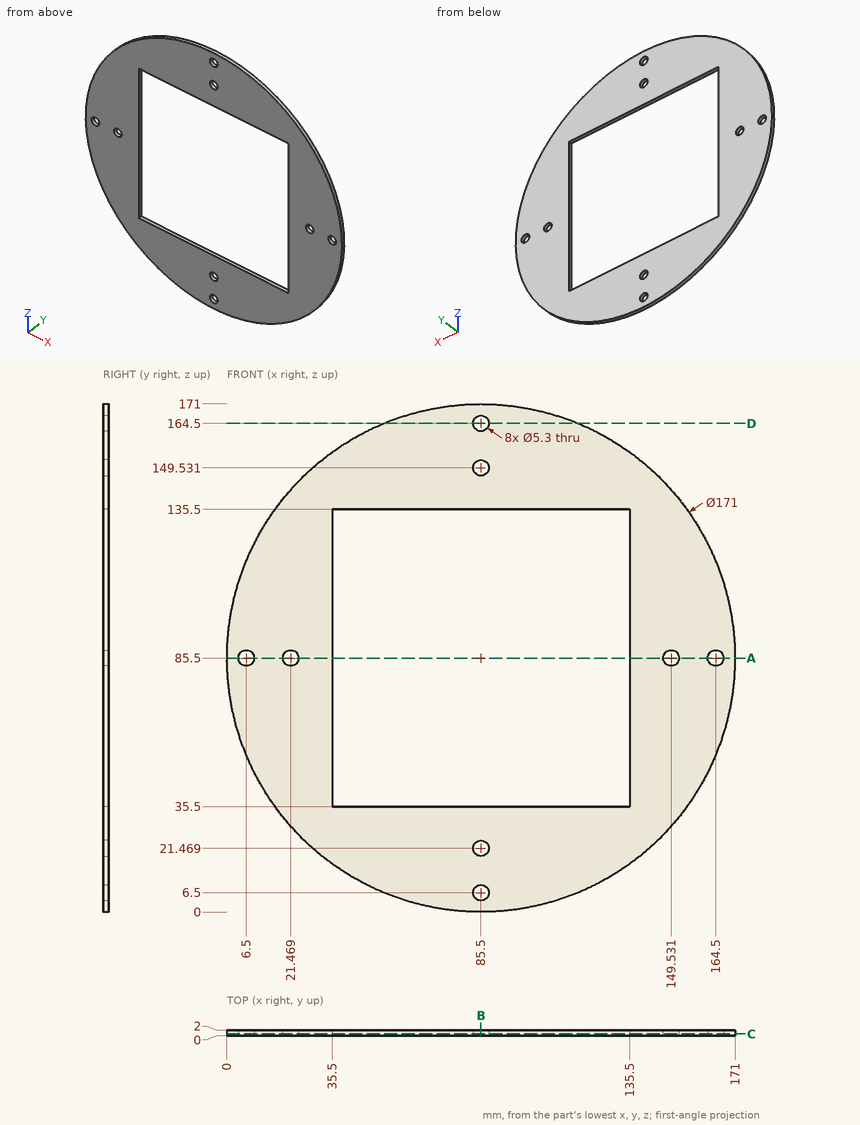
Input: dimensioned drawing with shaded views. Units: mm. Origin: part minimum x, y, z. Give positions to 0.01 mm unless a question says otherwise; leave off trailing zeros. Order: outer loops, then holes, each group sorted by start corner. A loop starts at its lowest first (then second) coordinate and runs counter-clockwise, first axis right, second up. Notation, with made-up numbers: (35, 57) -> (83, 57) arc R15 ccw to (83, 70) -> close; hole circle Ø4 at (-6.75, 65). An arc over 180 degrees is marked (long way). Answer as a JSON object with one key per item and string values.
Q1. First-contact query: pin 1 (0.6 mm diameter, centred on y = 0.5, z = 74, fed in from -X); pin 2 (1 mm diameter, centred on x = 152, y = 2, fed in from +Z); pin 3 (1 mm diameter, centred on y = 0.5, z = 134.5, fed in from +X); pin 4 (6 mm diameter, centred on x = 21.47, z = 85.5, fed in from +Y). Flat tips, straight axial feed; report the tip coordinate or a pass-through.
Entries:
{"pin 1": "stops at x = 0.74", "pin 2": "stops at z = 139.85", "pin 3": "stops at x = 155.91", "pin 4": "stops at y = 2"}
Q2. Material intervals for probe 1 along X at (y, z) = (0.7, 85.5); probe 2 along Z at (x, y) = (86, 0.1); probe 3 along X at (y, z) = (0.95, 100.5), sorted ascending.
Entries:
{"probe 1": "x = 0 to 3.85, 9.15 to 18.82, 24.12 to 35.5, 135.5 to 146.88, 152.18 to 161.85, 167.15 to 171", "probe 2": "z = 0 to 3.9, 9.1 to 18.87, 24.07 to 35.5, 135.5 to 146.93, 152.13 to 161.9, 167.1 to 171", "probe 3": "x = 1.33 to 35.5, 135.5 to 169.67"}
Q3. Section B-B (x = 85.5). Output: boundary loops of the cut face in (y, z).
Entries:
{"outline": "(0, 0) -> (2, 0) -> (2, 3.85) -> (0, 3.85) -> close; (0, 9.15) -> (2, 9.15) -> (2, 18.82) -> (0, 18.82) -> close; (0, 24.12) -> (2, 24.12) -> (2, 35.5) -> (0, 35.5) -> close; (0, 135.5) -> (2, 135.5) -> (2, 146.88) -> (0, 146.88) -> close; (0, 152.18) -> (2, 152.18) -> (2, 161.85) -> (0, 161.85) -> close; (0, 167.15) -> (2, 167.15) -> (2, 171) -> (0, 171) -> close"}
Q4. Section D-D (z = 164.5). Output: boundary loops of the cut face in (x, y).
Entries:
{"outline": "(52.8, 0) -> (82.85, 0) -> (82.85, 2) -> (52.8, 2) -> close; (88.15, 0) -> (118.2, 0) -> (118.2, 2) -> (88.15, 2) -> close"}
Q5. Section A-A (z = 85.5). Output: boundary loops of the cut face in (x, y).
Entries:
{"outline": "(0, 0) -> (3.85, 0) -> (3.85, 2) -> (0, 2) -> close; (9.15, 0) -> (18.82, 0) -> (18.82, 2) -> (9.15, 2) -> close; (24.12, 0) -> (35.5, 0) -> (35.5, 2) -> (24.12, 2) -> close; (135.5, 0) -> (146.88, 0) -> (146.88, 2) -> (135.5, 2) -> close; (152.18, 0) -> (161.85, 0) -> (161.85, 2) -> (152.18, 2) -> close; (167.15, 0) -> (171, 0) -> (171, 2) -> (167.15, 2) -> close"}
Q6. Section C-C (y = 0.7). State how many separate pieces and enclosed holes the cut face has, plus the area to 3 significant figures.
Entries:
{"separate pieces": "1", "enclosed holes": "9", "area": "12,800 mm^2"}
